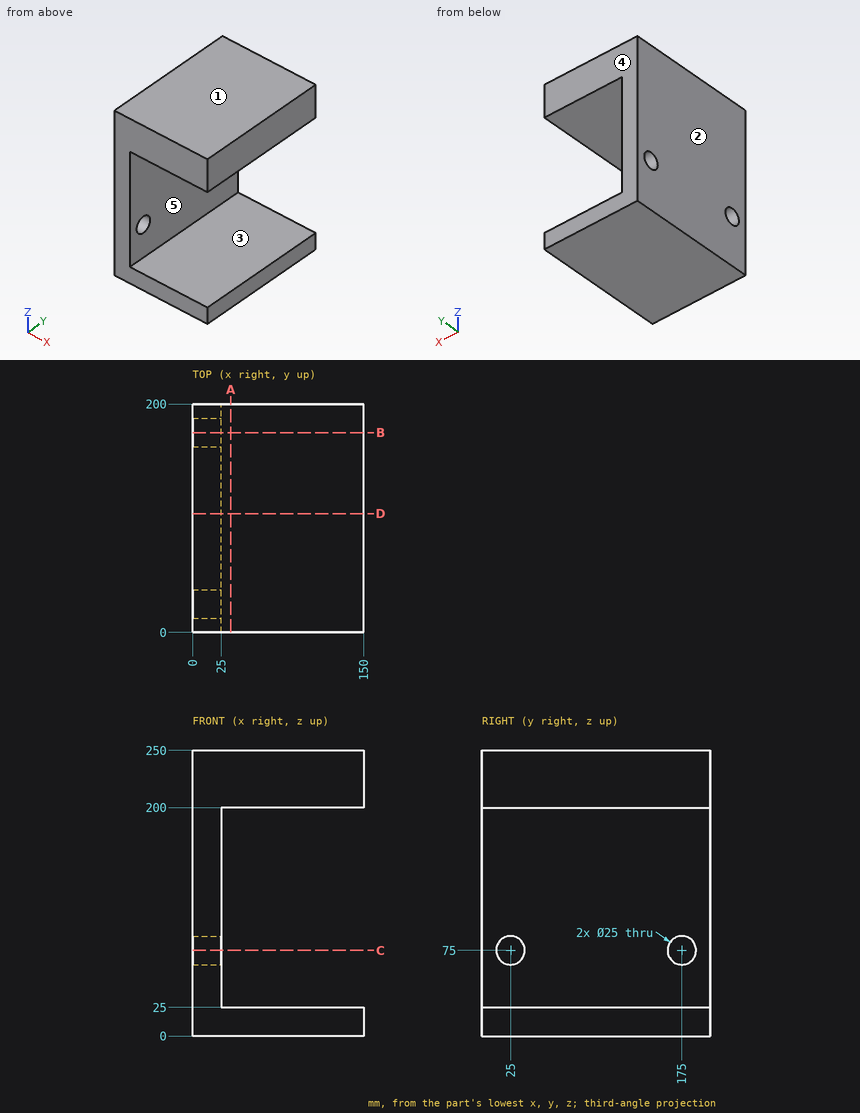
Geometry check sheet. Reference: drawing and pictorial views, mm from the part's lowest x, y, z. A direction names the side the tool comes from. Round coordinates to 2 decimals unless told otherwise and drop trailing zeros. Order: outer loops, then holes, each group sorted by start corner. A loop starts at its lowest first (then second) coordinate and runs counter-clockwise, first axis right, second up. Notation, with made-up numbers: (39.5, 82.5) - (98.5, 82.5) arc R16 ccw to (98.5, 113.5) - close; hole circle Ø11 at (87, -9.75). An arc over 180 degrees is marked (long way). One line per question, with ' | ' between items. Start each with the question number.
(1) Sectioned sample at B-B on y = 175. Record the cut outline in (x, z).
(2) Access from +Z, -Z, +X, -X, +Y, -Y to the whole of each face (thin tool, end or side, straight path). Record for the marked faces 4 and 5.
(3) Release check for a two-part mould opening along Z. For the marked faces 1, 2 and 3 record: released by +Z, released by -Z, zero draft, split by the parting line, or undercut.
(4) Sectioned sample at C-C on z = 75. Record the cut outline in (x, y).
(5) Thickness scan on L1, parallel to Y at x = 7, z = 75; L2, parallel to Z at x = 137.5, y = 59; L3, parallel to Z at x = 18, y = 175. Record the ranges inside material, lowest first. Write a range as [from, to].
(6) Sectioned sample at A-A on x = 33.5. Record the cut outline in (y, z), and give its area (3 significant figures).
(7) Sectioned sample at D-D on y = 104. Record the cut outline in (x, z), and give its area (3 significant figures).
Conclusion:
1) outline: (0, 0) - (150, 0) - (150, 25) - (25, 25) - (25, 62.5) - (0, 62.5) - close; (0, 87.5) - (25, 87.5) - (25, 200) - (150, 200) - (150, 250) - (0, 250) - close
2) face 4: +Z, -Z, +X, -X, +Y | face 5: +X, +Y, -Y
3) face 1: released by +Z | face 2: zero draft | face 3: undercut
4) outline: (0, 0) - (25, 0) - (25, 12.5) - (0, 12.5) - close; (0, 37.5) - (25, 37.5) - (25, 162.5) - (0, 162.5) - close; (0, 187.5) - (25, 187.5) - (25, 200) - (0, 200) - close
5) L1: y = [0, 12.5], [37.5, 162.5], [187.5, 200] | L2: z = [0, 25], [200, 250] | L3: z = [0, 62.5], [87.5, 250]
6) outline: (0, 0) - (200, 0) - (200, 25) - (0, 25) - close; (0, 200) - (200, 200) - (200, 250) - (0, 250) - close | area: 15,000 mm2
7) outline: (0, 0) - (150, 0) - (150, 25) - (25, 25) - (25, 200) - (150, 200) - (150, 250) - (0, 250) - close | area: 15,600 mm2
